Geometry: final body of the model. Coordinates: model frame, mm. Face numbers are marked on the shaded views. Round coordinates to 2 decimals unless told otherwise and drop trailing zeros. Write each loop counter-clockwise with the first axis right and the second up, starting at its lowest first coordinate (ties: lowest second). Pieces come first, ordered by that corner, then holes. Notation, with made-up numbers: (73.5, 30.25) - (95.5, 30.25) arc R16 ccw to (95.5, 54.25) - close; hole circle Ø10 at (88, -1). An arc over 180 degrees is marked (long way). Write each question's results on one line, items separated by ' | '.
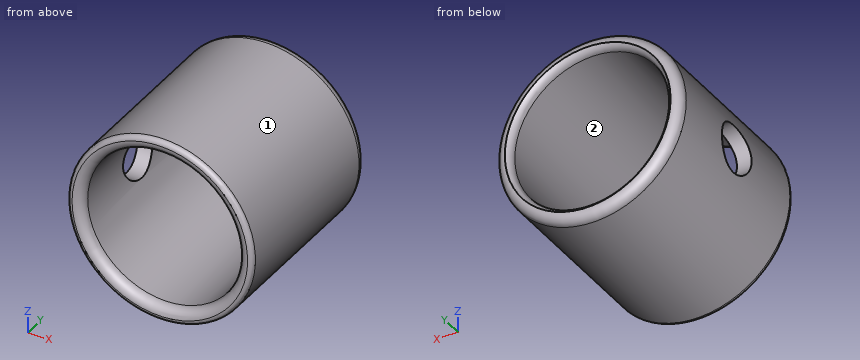
Autodesk Inventor part; units mm, degrees
ref_plane "YZ Plane" through (0, 0, 0) normal (1, 0, 0) x (0, 1, 0)
ref_plane "XZ Plane" through (0, 0, 0) normal (0, 1, 0) x (-1, 0, 0)
ref_plane "XY Plane" through (0, 0, 0) normal (0, 0, 1) x (1, 0, 0)
sketch "Sketch1" plane through (0, 0, 0) normal (0, 1, 0) x (-1, 0, 0)
  circle A0 centre (7.9604, -12.1069) radius 19
  circle A1 centre (7.9604, -12.1069) radius 16
  point P0 (0, 0)
  dimension "d0" = 38
  dimension "d1" = 32
extrude "Extrusion1" add sketch "Sketch1" along normal blind 38
fillet "Fillet1" radius 2 2 edges at (11.0396, 38, -12.1069) (8.0396, 38, -12.1069)
fillet "Fillet2" radius 1 1 edges at (11.0396, 0, -12.1069)
fillet "Fillet3" radius 2 1 edges at (8.0396, 0, -12.1069)
sketch "Sketch2" plane through (0, 0, 0) normal (1, 0, 0) x (0, 1, 0)
  line L0 (39.783, 8.7002) -> (-1.9245, -33.003)
  circle A0 centre (18.9293, -12.1514) radius 5
  point P0 (0, 0)
  dimension "d7" = 10
extrude "Extrusion2" cut sketch "Sketch2" against normal blind 38
properties part number "Bucha"
Q1. Ray query, line 1 along X through (y, z) = (28, -15.5); line 2 along X through (y, z) = (4.5, 1); line 3 along Z through (x, y) = (-10, 32.5). Return the intervals inside material, ascending.
Answer block:
line 1: -26.65 to -23.6, 7.68 to 10.73 | line 2: -21.72 to -17.14, 1.22 to 5.79 | line 3: -31 to -27.98, 3.76 to 6.78
Q2. Pin query (flat end, axial travel): pin 1 (1 mm diameter, centred on y = 11, z = -4.5, fed in from +X); pin 2 (8 mm diameter, centred on y = 11, z = -17, fed in from -X); pin 3 (1 mm diameter, centred on x = -8.5, y = 11, fed in from -Z); pin 4 (12 mm diameter, centred on x = -3, z = 2, fed in from -Y). Return the tip coordinate at first contact, or that it passes through.
Answer block:
pin 1: x = 9.66 | pin 2: x = -26.94 | pin 3: z = -31.11 | pin 4: y = 0
Q3. Mould query, pull axis X, two halves, no side actions, for the marked faces 1 and 2. Classes: pulls with the +X half, pulls with the -X half, needs draft (parallel to the pull), parting line crosses it, or undercut.
Answer block:
face 1: parting line crosses it | face 2: undercut
Q4. Section query B-B, the plane z = -11. Give the number of separate pieces and of enclosed holes in the cut face, plus the area to 3 significant figures.
Answer block:
separate pieces: 3 | enclosed holes: 0 | area: 194 mm2
Q5. Section query A-A, the plane y = 5. Return loops of the section in (x, z), plus the area to 3 significant figures.
Answer block:
outline: circle Ø38 at (-7.96, -12.11); hole circle Ø32 at (-7.96, -12.11) | area: 330 mm2
Q6. Section query C-C, the plane y = 21. Return loops of the section in (x, z).
Answer block:
outline: (-26.42, -7.6) - (-23.31, -7.6) arc R16 cw (long way) to (-23.29, -16.7) - (-26.4, -16.7) arc R19 ccw (long way) to start
